Read the model definition and answer for the solid it produces. Units are mm, in the model's axes. A direction names the side the tool comes from. Give positions to 0.01 mm unless a question says otherwise; leave off trailing zeros. Write each loop counter-clockwise with the first axis right and the second up, starting at its lowest first coordinate (ties: lowest second). Pieces come first, ordered by that corner, then holes. Notation, with made-up numbers: M 2.5,-24.75 L 40.5,-24.75 A12 ccw 40.5,-18.75 Z; hole C 45,12 d2. An arc over 180 degrees is marked long. Use a Markdown table: item, result. Add a question column.
Item 1: A cutting plane is placed at C-C on x = 72.5. Determine the outline of the cut face in (y, z), then the cut area to 3 significant figures.
Item 2: Given P1, Ø6, axis at x = 153, y = 92.5, coming from the -Z side; P2, Ø2, axis at x = 44.5, z = 23, coming from the +Y side; P3, Ø6, axis at x = 79.5, y = 71, coming from the +Z side, each flat-ended and moving along its own axis, determine where each tip first touches the part or whether it passes through.
Item 3: A cutting plane is placed at D-D on z = 10. Determine the outline of the cut face in (x, y).
Item 4: For faces 5 (the flat face through (6, 90, 12)), 6 (the flat face through (154, -10, 12)), 7 (the flat face through (79, 41, 6)), determine the directions among +Z, -Z, +X, -X, +Y, -Y from which every point of the face is accessible in a straight line to the end or side of a thin tool.
Item 5: Consider probe 1 along X at (y, z) = (71, 15); probe 2 along Y at (x, z) = (72, 19.5); probe 3 along X at (y, z) = (-7.5, 29). Determine where each line is inside the solid, lowest interval first. Write a range as [from, to].
Item 6: A cutting plane is placed at B-B on y = 58.5. Determine the outline of the cut face in (x, z), then the cut area to 3 significant figures.
Item 7: The mould has two halves that part along Y. Classify faces 1 (the flat face through (154, 100, 22)), 2 (the flat face through (154, -20, 22)), 3 (the flat face through (156, 40, 19)), 4 (the flat face through (12, -10, 22)): pulls with the +Y half, pulls with the -Y half, needs draft (parallel to the pull), parting line crosses it, or undercut.
Item 8: A cutting plane is placed at A-A on z = 20. Determine the outline of the cut face in (x, y).
from build123d import *

# Parameters (mm, degrees)
SKETCH_W     = 160
SKETCH_H     = 80
PAD_DEPTH    = 32
POCKET_DEPTH = 26
SKETCH002_W  = 12
SKETCH002_H  = 20
PAD001_DEPTH = 20
SKETCH003_W  = 12
SKETCH003_H  = 20
PAD002_DEPTH = 20


with BuildPart() as part:
    # Sketch → Pad (new body)
    with BuildSketch(Plane.XY):
        with Locations((80, 40)):
            Rectangle(SKETCH_W, SKETCH_H)
    extrude(amount=PAD_DEPTH)

    # Sketch001 (on Face6 of Pad) → Pocket (cut)
    with BuildSketch(Plane.XY.offset(32)):
        Polygon((8, 76), (4, 72), (4, 8), (8, 4), (152, 4), (156, 8), (156, 72), (152, 76), align=None)
    extrude(amount=-POCKET_DEPTH, mode=Mode.SUBTRACT)

    # Sketch002 (on Face6 of Pocket) → Pad001 (join)
    with BuildSketch(Plane.XZ):
        with Locations((154, 22)):
            Rectangle(SKETCH002_W, SKETCH002_H)
        with Locations((6, 22)):
            Rectangle(SKETCH002_W, SKETCH002_H)
    extrude(amount=PAD001_DEPTH)

    # Sketch003 (on Face1 of Pad001) → Pad002 (join)
    with BuildSketch(Plane(origin=(0, 80, 0), x_dir=(-1, 0, 0), z_dir=(0, 1, 0))):
        with Locations((-154, 22)):
            Rectangle(SKETCH003_W, SKETCH003_H)
        with Locations((-6, 22)):
            Rectangle(SKETCH003_W, SKETCH003_H)
    extrude(amount=PAD002_DEPTH)


solid = part.part
Filled in:
| question | item | result |
|---|---|---|
| 1 | outline | M 0,0 L 80,0 L 80,32 L 76,32 L 76,6 L 4,6 L 4,32 L 0,32 Z |
| 1 | area | 688 mm² |
| 2 | P1 | z = 12 |
| 2 | P2 | y = 80 |
| 2 | P3 | z = 6 |
| 3 | outline | M 0,0 L 160,0 L 160,80 L 0,80 Z; hole M 4,8 L 8,4 L 152,4 L 156,8 L 156,72 L 152,76 L 8,76 L 4,72 Z |
| 4 | face 5 | -Z, +X, -X, +Y |
| 4 | face 6 | -Z, +X, -X, -Y |
| 4 | face 7 | +Z |
| 5 | probe 1 | [0, 4], [156, 160] |
| 5 | probe 2 | [0, 4], [76, 80] |
| 5 | probe 3 | [0, 12], [148, 160] |
| 6 | outline | M 0,0 L 160,0 L 160,32 L 156,32 L 156,6 L 4,6 L 4,32 L 0,32 Z |
| 6 | area | 1,170 mm² |
| 7 | face 1 | pulls with the +Y half |
| 7 | face 2 | pulls with the -Y half |
| 7 | face 3 | undercut |
| 7 | face 4 | needs draft |
| 8 | outline | M 0,-20 L 12,-20 L 12,0 L 148,0 L 148,-20 L 160,-20 L 160,100 L 148,100 L 148,80 L 12,80 L 12,100 L 0,100 Z; hole M 4,8 L 8,4 L 152,4 L 156,8 L 156,72 L 152,76 L 8,76 L 4,72 Z |
